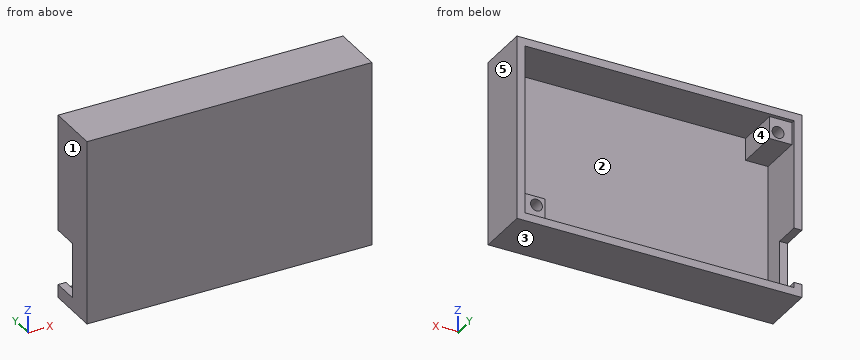
from build123d import *

# Parameters (mm, degrees)
SKETCH1_W               = 108.5
SKETCH1_H               = 70.5
BOSS_EXTRUDE1_DEPTH     = 20
SKETCH2_W               = 102.5
SKETCH2_H               = 64.5
CUT_EXTRUDE1_DEPTH      = 18
SKETCH3_W               = 8.5
SKETCH3_H               = 8.5
BOSS_EXTRUDE2_DEPTH     = 16.5
SKETCH4_R               = 2.25
CUT_EXTRUDE2_DEPTH      = 15
SKETCH7_W               = 21
SKETCH7_H               = 10
CUT_EXTRUDE5_DEPTH      = 8
SKETCH8_W               = 8.5
SKETCH8_H               = 8.5
BOSS_EXTRUDE3_DEPTH     = 16.5
CUT_EXTRUDE6_DEPTH      = 13
CUT_EXTRUDE6_DEPTH_BACK = 15
SKETCH9_R               = 2.25


with BuildPart() as part:
    # Sketch1 → Boss-Extrude1 (new body)
    with BuildSketch(Plane(origin=(0, 0, 0), x_dir=(1, 0, 0), z_dir=(0, 1, 0))):
        Rectangle(SKETCH1_W, SKETCH1_H)
    extrude(amount=BOSS_EXTRUDE1_DEPTH)

    # Sketch2 → Cut-Extrude1 (cut)
    with BuildSketch(Plane(origin=(0, 20, 0), x_dir=(1, 0, 0), z_dir=(0, 1, 0))):
        Rectangle(SKETCH2_W, SKETCH2_H)
    extrude(amount=-CUT_EXTRUDE1_DEPTH, mode=Mode.SUBTRACT)

    # Sketch3 → Boss-Extrude2 (add)
    with BuildSketch(Plane(origin=(0, 2, 0), x_dir=(1, 0, 0), z_dir=(0, 1, 0))):
        with Locations((-47, -28)):
            Rectangle(SKETCH3_W, SKETCH3_H)
    extrude(amount=BOSS_EXTRUDE2_DEPTH)

    # Sketch4 → Cut-Extrude2 (cut)
    with BuildSketch(Plane(origin=(0, 18.5, 0), x_dir=(1, 0, 0), z_dir=(0, 1, 0))):
        with Locations(Location((-46, -27, 0), (0, 0, 270))):
            Circle(SKETCH4_R)
    extrude(amount=-CUT_EXTRUDE2_DEPTH, mode=Mode.SUBTRACT)

    # Sketch7 → Cut-Extrude5 (cut)
    with BuildSketch(Plane(origin=(-51.25, 0, 0), x_dir=(0, 0, -1), z_dir=(1, 0, 0))):
        with Locations((19.75, 15)):
            Rectangle(SKETCH7_W, SKETCH7_H)
    extrude(amount=-CUT_EXTRUDE5_DEPTH, mode=Mode.SUBTRACT)

    # Sketch8 → Boss-Extrude3 (add)
    with BuildSketch(Plane(origin=(0, 2, 0), x_dir=(1, 0, 0), z_dir=(0, 1, 0))):
        with Locations((47, 28)):
            Rectangle(SKETCH8_W, SKETCH8_H)
    extrude(amount=BOSS_EXTRUDE3_DEPTH)

    # Sketch9 → Cut-Extrude6 (cut, two sides: drawn at the far end of the back side and taken through both)
    with BuildSketch(Plane(origin=(0, 18.5, 0), x_dir=(1, 0, 0), z_dir=(0, 1, 0)).offset(-CUT_EXTRUDE6_DEPTH_BACK)):
        with Locations(Location((46, 27, 0), (0, 0, 90))):
            Circle(SKETCH9_R)
    extrude(amount=CUT_EXTRUDE6_DEPTH + CUT_EXTRUDE6_DEPTH_BACK, mode=Mode.SUBTRACT)


solid = part.part
For this review, take the finished solid that the model builds, in its own axes (mm). Face numbers are marked on the shaded views. A direction names the side the tool comes from. Round coordinates to 2 decimals unless told otherwise and drop trailing zeros. Write each loop counter-clockwise with the first axis right and the second up, starting at its lowest first coordinate (ties: lowest second). Pieces come first, ordered by that corner, then holes. Notation, with made-up numbers: M 71.25,70.25 L 97.25,70.25 A18 ccw 97.25,81.25 Z; hole C 32.5,-30.75 d7. An arc over 180 degrees is marked long. Write item = value, one per line. Start each with the question number.
(1) For line 1 along Z through (x, y) = (46, 10); line 2 along X through (y, z) = (13.5, 27); line 3 along Z through (x, y) = (21, 18.5), list the stretches that pass through material, from the lowest coordinate up.
(2) For the marked faces 1 and 2, list the 3-axis set-ups (+Z, -Z, +X, -X, +Y, -Y) from which the entire face can be reached by the end or side of a thin tool; tool diameter is ignored.
(3) We need section A-A (y = 7.75). Give the boundary of the cut face in (x, z).
(4) Clearance check with flat-ended pins moving along their axes: pin 1 Ø1.5 at (x, z) = (-53, -17) entering from +Y; pin 2 Ø1 at (y, z) = (16.5, -17) entering from -X; pin 3 Ø2 at (x, z) = (-42.5, 8.5) entering from +Y. State where each tip first meets the part, or that it passes through.
(5) We need section C-C (z = 27). Give the boundary of the cut face in (x, y), then the cut area to 3 significant figures.
(6) We need section B-B (x = -46). Give the boundary of the cut face in (y, z), then the cut area to 3 significant figures.
(7) We need section D-D (x = 26.5). Give the boundary of the cut face in (y, z).
(8) The part is to be moulded in two halves that separate along X. For the marked faces 3, 4 and 5, say which applies: +X half, -X half, draft (parallel to the pull), parting line (faces both ways), or undercut.
Results found:
q1.line_1 = -35.25 to -29.25, -24.75 to -23.75, 32.25 to 35.25
q1.line_2 = -54.25 to -48.25, -43.75 to -42.75, 51.25 to 54.25
q1.line_3 = -35.25 to -32.25, 32.25 to 35.25
q2.face_1 = +Z, -Z, -X, +Y, -Y
q2.face_2 = +Y
q3.outline = M -54.25,-35.25 L 54.25,-35.25 L 54.25,35.25 L -54.25,35.25 Z; hole M -51.25,-32.25 L 42.75,-32.25 L 42.75,-23.75 L 51.25,-23.75 L 51.25,32.25 L -42.75,32.25 L -42.75,23.75 L -51.25,23.75 Z; hole C -46,27 d4.5; hole C 46,-27 d4.5
q4.pin_1 = 10
q4.pin_2 = 51.25
q4.pin_3 = 2
q5.outline = M -54.25,0 L 54.25,0 L 54.25,20 L 51.25,20 L 51.25,2 L -42.75,2 L -42.75,18.5 L -43.75,18.5 L -43.75,3.5 L -48.25,3.5 L -48.25,18.5 L -51.25,18.5 L -51.25,20 L -54.25,20 Z
q5.area = 398 mm²
q6.outline = M 0,-35.25 L 20,-35.25 L 20,-32.25 L 2,-32.25 L 2,23.75 L 18.5,23.75 L 18.5,24.75 L 3.5,24.75 L 3.5,29.25 L 18.5,29.25 L 18.5,32.25 L 20,32.25 L 20,35.25 L 0,35.25 Z
q6.area = 322 mm²
q7.outline = M 0,-35.25 L 20,-35.25 L 20,-32.25 L 2,-32.25 L 2,32.25 L 20,32.25 L 20,35.25 L 0,35.25 Z
q8.face_3 = draft
q8.face_4 = undercut
q8.face_5 = +X half
